```python
from build123d import *

# Parameters (mm, degrees)
SKETCH1_W           = 22.6
SKETCH1_H           = 12.4
BOSS_EXTRUDE1_DEPTH = 22.3
SKETCH2_W           = 12.4
SKETCH2_H           = 2.4
BOSS_EXTRUDE2_DEPTH = 5
BOSS_EXTRUDE4_DEPTH = 4.3
SKETCH7_R           = 2.5
BOSS_EXTRUDE5_DEPTH = 3.3


with BuildPart() as part:
    # Sketch1 → Boss-Extrude1 (new body)
    with BuildSketch(Plane(origin=(0, 0, 0), x_dir=(1, 0, 0), z_dir=(0, 1, 0))):
        Rectangle(SKETCH1_W, SKETCH1_H)
    extrude(amount=BOSS_EXTRUDE1_DEPTH)

    # Sketch2 → Boss-Extrude2 (add)
    with BuildSketch(Plane(origin=(11.3, 0, 0), x_dir=(0, 0, -1), z_dir=(1, 0, 0))):
        with Locations((0, 16.85)):
            Rectangle(SKETCH2_W, SKETCH2_H)
    extrude(amount=BOSS_EXTRUDE2_DEPTH)

    # Sketch6 → Boss-Extrude4 (add)
    with BuildSketch(Plane(origin=(0, 22.3, 0), x_dir=(1, 0, 0), z_dir=(0, 1, 0))):
        with BuildLine():
            ThreePointArc((0.966666667, -1.278888406), (2.5, 0), (0.966666667, 1.278888406))
            ThreePointArc((0.966666667, 1.278888406), (-11.3, 0), (0.966666667, -1.278888406))
        make_face()
    extrude(amount=BOSS_EXTRUDE4_DEPTH)

    # Sketch7 → Boss-Extrude5 (add)
    with BuildSketch(Plane(origin=(0, 26.6, 0), x_dir=(1, 0, 0), z_dir=(0, 1, 0))):
        with Locations((-5.1, 0)):
            Circle(SKETCH7_R)
    extrude(amount=BOSS_EXTRUDE5_DEPTH)


solid = part.part
```
Geometry: final body of the model. Coordinates: model frame, mm. A direction names the side the tool comes from. Coordinates: 2 decimals unless noted, no trailing zeros. Order: outer loops, then holes, each group sorted by start corner. A loop starts at its lowest first (then second) coordinate and runs counter-clockwise, first axis right, second up. Notation, with made-up numbers: (8, 26.25) - (27, 26.25) arc R26 ccw to (27, 40.25) - close; hole circle Ø4 at (-26, -38). An arc over 180 degrees is marked (long way). Return JSON: item names as keys, results as strings. Group by question number.
1. Material intervals for line 1 along X through (y, z) = (5.5, -2); line 2 along Y through (x, z) = (11.25, -2.25); line 3 along Y through (x, z) = (-8.75, -1.75), sorted ascending. Write a range as [from, to].
2. Pin query (flat end, axial travel): pin 1 (6 mm diameter, centred on x = -1.5, z = 2, fed in from +Y); pin 2 (5 mm diameter, centred on y = 26.5, z = -4, fed in from +X); pin 3 (4 mm diameter, centred on x = 14, z = 1, fed in from -Y); pin 4 (2.5 mm diameter, centred on x = 13, z = 1, fed in from +Y). Return the tip coordinate at first contact, or that it passes through.
3. Cut plane D-D (x = 12.5). Output: boundary loops of the cut face in (y, z), plus the area to 3 significant figures.
4. Cut plane C-C (y = 6.5). Output: boundary loops of the cut face in (x, z), plus the area to 3 significant figures.
5. Cut plane B-B (z = -4). Output: boundary loops of the cut face in (x, y), plus the area to 3 significant figures.
6. Set-up query: faces 1 (the face through (14, 18.05, 0)), 2 (the face through (-4, 26.6, 3)), 3 (the face through (-10, 22.3, 5)). Return all of +Z, -Z, +X, -X, +Y, -Y with unobstructed straight access to the full face (end or side cutting, diameter ignored); none if empty.
7. Cut plane A-A (x = -0.5). Output: boundary loops of the cut face in (y, z), plus the area to 3 significant figures.
Resolved:
{
 "1": {"line 1": "x = [-11.3, 11.3]", "line 2": "y = [0, 22.3]", "line 3": "y = [0, 26.6]"},
 "2": {"pin 1": "stops at y = 29.9", "pin 2": "stops at x = 0.92", "pin 3": "stops at y = 15.65", "pin 4": "stops at y = 18.05"},
 "3": {"outline": "(15.65, -6.2) - (18.05, -6.2) - (18.05, 6.2) - (15.65, 6.2) - close", "area": "29.8 mm²"},
 "4": {"outline": "(-11.3, -6.2) - (11.3, -6.2) - (11.3, 6.2) - (-11.3, 6.2) - close", "area": "280 mm²"},
 "5": {"outline": "(-11.3, 0) - (11.3, 0) - (11.3, 15.65) - (16.3, 15.65) - (16.3, 18.05) - (11.3, 18.05) - (11.3, 22.3) - (-0.36, 22.3) - (-0.36, 26.6) - (-9.84, 26.6) - (-9.84, 22.3) - (-11.3, 22.3) - close", "area": "557 mm²"},
 "6": {"face 1": "+Z, -Z, +X, +Y", "face 2": "+Y", "face 3": "+Z, -X, +Y"},
 "7": {"outline": "(0, -6.2) - (22.3, -6.2) - (22.3, -4.16) - (26.6, -4.16) - (26.6, 4.16) - (22.3, 4.16) - (22.3, 6.2) - (0, 6.2) - close", "area": "312 mm²"}
}
